```python
from build123d import *

# Parameters (mm, degrees)
F3_DEPTH = 12.5


with BuildPart() as f1:
    # F0 (on Front) → F1 (revolve)
    with BuildSketch(Plane.XZ):
        with BuildLine():
            ThreePointArc((-18.0916087155, 2.4896269549), (-9.0697101385, 3.4763084496), (0, 3.8057812268))
            Line((0, 3.8057812268), (0, 15.685))
            ThreePointArc((0, 15.685), (-7.408626068, 14.1810641227), (-13.6443996575, 9.9073431353))
            ThreePointArc((-13.6443996575, 9.9073431353), (-16.295679955, 6.4548932852), (-18.0916087155, 2.4896269549))
        make_face()
        with BuildLine():
            ThreePointArc((-21.3346085291, 1.9716631865), (-19.7148097422, 2.2412958765), (-18.0916087155, 2.4896269549))
            ThreePointArc((-18.0916087155, 2.4896269549), (-16.295679955, 6.4548932852), (-13.6443996575, 9.9073431353))
            Line((-13.6443996575, 9.9073431353), (-20.3248404986, 3.0136629614))
            Line((-20.3248404986, 3.0136629614), (-21.3346085291, 1.9716631865))
        make_face()
        with BuildLine():
            ThreePointArc((-22.7378459416, 1.7203465229), (-25.8145491381, 1.1111738013), (-28.875, 0.425))
            Line((-28.875, 0.425), (-18.6282688407, 0.425))
            ThreePointArc((-18.6282688407, 0.425), (-18.3889375183, 1.464851143), (-18.0916087155, 2.4896269549))
            ThreePointArc((-18.0916087155, 2.4896269549), (-19.7148097422, 2.2412958765), (-21.3346085291, 1.9716631865))
            ThreePointArc((-21.3346085291, 1.9716631865), (-22.0365855065, 1.848005277), (-22.7378459416, 1.7203465229))
        make_face()
        Polygon((-28.875, -0.425), (0, -0.425), (0, 0), (0, 0.425), (-18.6282688407, 0.425), (-28.875, 0.425), align=None)
        with BuildLine():
            ThreePointArc((-20.3248404986, 3.0136629614), (-21.4306013049, 2.1790454907), (-22.7378459416, 1.7203465229))
            ThreePointArc((-22.7378459416, 1.7203465229), (-22.0365855065, 1.848005277), (-21.3346085291, 1.9716631865))
            Line((-21.3346085291, 1.9716631865), (-20.3248404986, 3.0136629614))
        make_face()
        with BuildLine():
            Line((-18.6282688407, 0.425), (0, 0.425))
            Line((0, 0.425), (0, 3.8057812268))
            ThreePointArc((0, 3.8057812268), (-9.0697101385, 3.4763084496), (-18.0916087155, 2.4896269549))
            ThreePointArc((-18.0916087155, 2.4896269549), (-18.3889375183, 1.464851143), (-18.6282688407, 0.425))
        make_face()
    revolve(axis=Axis((0, 0, 10.397832983), (0, 0, 1)))

    # F2 (on Right) → F3 (cut, symmetric)
    with BuildSketch(Plane.YZ):
        Polygon((-34.8162702815, 14.675), (27.6827993542, 14.675), (-3.9353072157, 26.7957725373), (-36.1574023472, 14.675), align=None)
    extrude(amount=F3_DEPTH, both=True, mode=Mode.SUBTRACT)


solid = f1.part
```
The listing builds one solid part. Answer for the finished solid, in the listing's coordinates (mm). Give positions to 0.01 mm unless a question says otherwise; leave off trailing zeros. Order: outer loops, then holes, each group sorted by start corner. A loop starts at its lowest first (then second) coordinate and runs counter-clockwise, first axis right, second up. Notation, with made-up numbers: (3.25, 29.5) - (36.25, 29.5) arc R25 cw to (36.25, 59.5) - close; hole circle Ø9 at (82.25, 20.5). An arc over 180 degrees is marked (long way). Use one line per item in the form item = value. Start each with the question number.
(1) Consider line 1 (Z direction, x = -11, y = 8) (1 decimal); line 2 (Z direction, x = -9.5, y = 13) (3 decimals); line 3 (X direction, y = -9, z = 4.75). Determine where each line is inside the solid, lowest interval first. Write a range as from..to.
(2) A cutting plane is placed at A-A, the plane x = 0. Write down the section's boundary in (y, z) (3 decimals), then the cut area to 3 significant figures.
(3) Flat-ended cylindrical pins translate along their axes: pin 1 Ø6 at (y, z) = (14, 11.5) entering from -X; pin 2 Ø3 at (x, y) = (9, 19) entering from +Z; pin 3 Ø6 at (y, z) = (21, 2.5) entering from -X. Find the tip coordinate at first contact, or state that the pin passes through.
(4) A cutting plane is placed at C-C, the plane z = 7.25. Write down the section's boundary in (x, y), then the cut area to 3 significant figures.
Ans:
q1.line_1 = -0.4..10
q1.line_2 = -0.425..7.372
q1.line_3 = -16.33..16.33
q2.outline = (-28.875, -0.425) - (28.875, -0.425) - (28.875, 0.425) arc R125 ccw to (22.738, 1.72) arc R4.5 cw to (20.325, 3.014) - (13.644, 9.907) arc R19 ccw to (6.112, 14.675) - (-6.112, 14.675) arc R19 ccw to (-13.644, 9.907) - (-20.325, 3.014) arc R4.5 cw to (-22.738, 1.72) arc R125 ccw to (-28.875, 0.425) - close
q2.area = 506 mm^2
q3.pin_1 = -7.72
q3.pin_2 = 3.84
q3.pin_3 = -21.89
q4.outline = circle Ø32.44 at (0, 0)
q4.area = 826 mm^2
